Build history of the part. All positions in model axes, mm. A direction names the side the tool comes from. Coordinates: 2 decimals unless noted, no trailing zeros. Loops run counter-clockwise (first coordinate to the right, second up) from the corner with the lowest first, then second, coordinate; pieces in that order, holes last.
Item 1: Cut at B-B (x = -25). List the corners of the cut face in (y, z), and give its area (3 significant figures).
Item 2: Mould opens along Y. For faces 4 (the face through (-1, 4.5, 5)), 5 (the face through (92.5, 58.04, -0.16)), 6 (the face through (0, 98.1, -2)), 7 (the face through (-60.019, 87.575, -1.584)) say: released by +Y, released by -Y, zero draft, split by the parting line, or undercut.
Item 3: Cut at C-C (y = 65). List the corners of the cut face in (x, z).
Item 4: Cut at D-D (x = 60). List the corners of the cut face in (y, z), and give its area (3 significant figures).
Item 5: Drill centre lines: line 1 along Y through (x, z) = (36, -2.5); line 2 along X through (y, z) = (74, 4.25); line 3 along X through (y, z) = (64, -3.5). Where is each one in solid material? Low to high.
Item 6: Flat gauge pins, fed straight in: pin 1 (6 mm diameter, centred on x = 9, z = -3.5, fed in from -Y); pin 2 (4.5 mm diameter, centred on y = 60, z = -4.5, fed in from -X); pin 3 (3 mm diameter, centred on y = 86.5, z = 3.5, fed in from +X). Where does each tip first touch, or does it go through?
Item 7: 3-axis set-ups, long thin cutter, end or side, ignore diameter. For faces 1 (the face through (59.475, 88.119, -1.584)), 2 (the face through (0, 93.1, 0)), 3 (the face through (-78, 105, -7.5)): which of +Z, -Z, +X, -X, +Y, -Y reach the whole face in a straight line?
Item 8: Cut at A-A (z = 0). List the corners of the cut face in (x, y), and give its area (3 significant figures).
from build123d import *

# Parameters (mm, degrees)
BOSS_EXTRUDE1_DEPTH = 117.6
CUT_EXTRUDE4_DEPTH  = 12
CUT_EXTRUDE6_DEPTH  = 151.36957804
CUT_EXTRUDE7_DEPTH  = 4.5
CUT_EXTRUDE8_START  = 113.1
CUT_EXTRUDE8_DEPTH  = 4.5
CUT_EXTRUDE9_DEPTH  = 4.5
CUT_EXTRUDE10_START = 113.1
CUT_EXTRUDE10_DEPTH = 4.5


with BuildPart() as part:
    # Sketch2 → Boss-Extrude1 (new body)
    with BuildSketch(Plane(origin=(0, 0, 0), x_dir=(1, 0, 0), z_dir=(0, 1, 0))):
        with BuildLine():
            Line((85, -7.5), (-85, -7.5))
            ThreePointArc((-85, -7.5), (-92.5, 0), (-85, 7.5))
            Line((-85, 7.5), (85, 7.5))
            ThreePointArc((85, 7.5), (92.5, 0), (85, -7.5))
        make_face()
    extrude(amount=BOSS_EXTRUDE1_DEPTH)

    # Sketch3 → Cut-Extrude4 (cut)
    with BuildSketch(Plane(origin=(0, 0, -7.5), x_dir=(-1, 0, 0), z_dir=(0, 0, -1))):
        with BuildLine():
            Line((-50, 113.1), (50, 113.1))
            ThreePointArc((50, 113.1), (74.748737342, 102.848737342), (85, 78.1))
            Line((85, 78.1), (85, 39.5))
            ThreePointArc((85, 39.5), (74.748737342, 14.751262658), (50, 4.5))
            Line((50, 4.5), (-50, 4.5))
            ThreePointArc((-50, 4.5), (-74.748737342, 14.751262658), (-85, 39.5))
            Line((-85, 39.5), (-85, 78.1))
            ThreePointArc((-85, 78.1), (-74.748737342, 102.848737342), (-50, 113.1))
        make_face()
        with BuildLine():
            Line((-70, 63.1), (-70, 54.5))
            ThreePointArc((-70, 54.5), (-59.748737342, 29.751262658), (-35, 19.5))
            Line((-35, 19.5), (35, 19.5))
            ThreePointArc((35, 19.5), (59.748737342, 29.751262658), (70, 54.5))
            Line((70, 54.5), (70, 63.1))
            ThreePointArc((70, 63.1), (59.748737342, 87.848737342), (35, 98.1))
            Line((35, 98.1), (-35, 98.1))
            ThreePointArc((-35, 98.1), (-59.748737342, 87.848737342), (-70, 63.1))
        make_face(mode=Mode.SUBTRACT)
    extrude(amount=-CUT_EXTRUDE4_DEPTH, mode=Mode.SUBTRACT)

    # Sketch6 → Cut-Extrude6 (cut, through all)
    with BuildSketch(Plane(origin=(0, 0, -7.5), x_dir=(-1, 0, 0), z_dir=(0, 0, -1))):
        with BuildLine():
            Line((-35, 24.5), (35, 24.5))
            ThreePointArc((35, 24.5), (56.213203436, 33.286796564), (65, 54.5))
            Line((65, 54.5), (65, 63.1))
            ThreePointArc((65, 63.1), (56.213203436, 84.313203436), (35, 93.1))
            Line((35, 93.1), (-35, 93.1))
            ThreePointArc((-35, 93.1), (-56.213203436, 84.313203436), (-65, 63.1))
            Line((-65, 63.1), (-65, 54.5))
            ThreePointArc((-65, 54.5), (-56.213203436, 33.286796564), (-35, 24.5))
        make_face()
    extrude(amount=-CUT_EXTRUDE6_DEPTH, mode=Mode.SUBTRACT)

    # Sketch2_6 → Cut-Extrude7 (cut)
    with BuildSketch(Plane(origin=(0, 0, 0), x_dir=(1, 0, 0), z_dir=(0, 1, 0))):
        with BuildLine():
            Line((-8.2248772, -2.5), (8.2248772, -2.5))
            Line((8.2248772, -2.5), (15.34156858, -1.994983292))
            ThreePointArc((15.34156858, -1.994983292), (17.2, 0), (15.34156858, 1.994983292))
            Line((15.34156858, 1.994983292), (1.88348082, 2.95))
            ThreePointArc((1.88348082, 2.95), (0, 3.5), (-1.88348082, 2.95))
            Line((-1.88348082, 2.95), (-15.34156858, 1.994983292))
            ThreePointArc((-15.34156858, 1.994983292), (-17.2, 0), (-15.34156858, -1.994983292))
            Line((-15.34156858, -1.994983292), (-8.2248772, -2.5))
        make_face()
        with BuildLine():
            Line((1.88348082, -2.95), (8.2248772, -2.5))
            Line((8.2248772, -2.5), (-8.2248772, -2.5))
            Line((-8.2248772, -2.5), (-1.88348082, -2.95))
            ThreePointArc((-1.88348082, -2.95), (0, -3.5), (1.88348082, -2.95))
        make_face()
    extrude(amount=CUT_EXTRUDE7_DEPTH, mode=Mode.SUBTRACT)

    # Sketch2_7 → Cut-Extrude8 (cut)
    with BuildSketch(Plane(origin=(0, 0, 0), x_dir=(1, 0, 0), z_dir=(0, 1, 0)).offset(CUT_EXTRUDE8_START)):
        with BuildLine():
            Line((-8.2248772, -2.5), (8.2248772, -2.5))
            Line((8.2248772, -2.5), (15.34156858, -1.994983292))
            ThreePointArc((15.34156858, -1.994983292), (17.2, 0), (15.34156858, 1.994983292))
            Line((15.34156858, 1.994983292), (1.88348082, 2.95))
            ThreePointArc((1.88348082, 2.95), (0, 3.5), (-1.88348082, 2.95))
            Line((-1.88348082, 2.95), (-15.34156858, 1.994983292))
            ThreePointArc((-15.34156858, 1.994983292), (-17.2, 0), (-15.34156858, -1.994983292))
            Line((-15.34156858, -1.994983292), (-8.2248772, -2.5))
        make_face()
        with BuildLine():
            Line((1.88348082, -2.95), (8.2248772, -2.5))
            Line((8.2248772, -2.5), (-8.2248772, -2.5))
            Line((-8.2248772, -2.5), (-1.88348082, -2.95))
            ThreePointArc((-1.88348082, -2.95), (0, -3.5), (1.88348082, -2.95))
        make_face()
    extrude(amount=CUT_EXTRUDE8_DEPTH, mode=Mode.SUBTRACT)

    # Sketch2_8 → Cut-Extrude9 (cut)
    with BuildSketch(Plane(origin=(0, 0, 0), x_dir=(1, 0, 0), z_dir=(0, 1, 0))):
        with BuildLine():
            Line((85, -2.5), (85, 7.5))
            Line((85, 7.5), (-85, 7.5))
            Line((-85, 7.5), (-85, -2.5))
            Line((-85, -2.5), (-8.2248772, -2.5))
            Line((-8.2248772, -2.5), (-15.34156858, -1.994983292))
            ThreePointArc((-15.34156858, -1.994983292), (-17.2, 0), (-15.34156858, 1.994983292))
            Line((-15.34156858, 1.994983292), (-1.88348082, 2.95))
            ThreePointArc((-1.88348082, 2.95), (0, 3.5), (1.88348082, 2.95))
            Line((1.88348082, 2.95), (15.34156858, 1.994983292))
            ThreePointArc((15.34156858, 1.994983292), (17.2, 0), (15.34156858, -1.994983292))
            Line((15.34156858, -1.994983292), (8.2248772, -2.5))
            Line((8.2248772, -2.5), (85, -2.5))
        make_face()
        with BuildLine():
            Line((70, -7.5), (85, -7.5))
            ThreePointArc((85, -7.5), (92.5, 0), (85, 7.5))
            Line((85, 7.5), (85, -2.5))
            Line((85, -2.5), (8.2248772, -2.5))
            Line((8.2248772, -2.5), (1.88348082, -2.95))
            ThreePointArc((1.88348082, -2.95), (0, -3.5), (-1.88348082, -2.95))
            Line((-1.88348082, -2.95), (-8.2248772, -2.5))
            Line((-8.2248772, -2.5), (-85, -2.5))
            Line((-85, -2.5), (-85, 7.5))
            ThreePointArc((-85, 7.5), (-92.5, 0), (-85, -7.5))
            Line((-85, -7.5), (-70, -7.5))
            Line((-70, -7.5), (-55, -7.5))
            Line((-55, -7.5), (55, -7.5))
            Line((55, -7.5), (70, -7.5))
        make_face()
        with BuildLine():
            Line((1.88348082, -2.95), (8.2248772, -2.5))
            Line((8.2248772, -2.5), (-8.2248772, -2.5))
            Line((-8.2248772, -2.5), (-1.88348082, -2.95))
            ThreePointArc((-1.88348082, -2.95), (0, -3.5), (1.88348082, -2.95))
        make_face()
    extrude(amount=CUT_EXTRUDE9_DEPTH, mode=Mode.SUBTRACT)

    # Sketch2_9 → Cut-Extrude10 (cut)
    with BuildSketch(Plane(origin=(0, 0, 0), x_dir=(1, 0, 0), z_dir=(0, 1, 0)).offset(CUT_EXTRUDE10_START)):
        with BuildLine():
            Line((85, -2.5), (85, 7.5))
            Line((85, 7.5), (-85, 7.5))
            Line((-85, 7.5), (-85, -2.5))
            Line((-85, -2.5), (-8.2248772, -2.5))
            Line((-8.2248772, -2.5), (-15.34156858, -1.994983292))
            ThreePointArc((-15.34156858, -1.994983292), (-17.2, 0), (-15.34156858, 1.994983292))
            Line((-15.34156858, 1.994983292), (-1.88348082, 2.95))
            ThreePointArc((-1.88348082, 2.95), (0, 3.5), (1.88348082, 2.95))
            Line((1.88348082, 2.95), (15.34156858, 1.994983292))
            ThreePointArc((15.34156858, 1.994983292), (17.2, 0), (15.34156858, -1.994983292))
            Line((15.34156858, -1.994983292), (8.2248772, -2.5))
            Line((8.2248772, -2.5), (85, -2.5))
        make_face()
        with BuildLine():
            Line((70, -7.5), (85, -7.5))
            ThreePointArc((85, -7.5), (92.5, 0), (85, 7.5))
            Line((85, 7.5), (85, -2.5))
            Line((85, -2.5), (8.2248772, -2.5))
            Line((8.2248772, -2.5), (1.88348082, -2.95))
            ThreePointArc((1.88348082, -2.95), (0, -3.5), (-1.88348082, -2.95))
            Line((-1.88348082, -2.95), (-8.2248772, -2.5))
            Line((-8.2248772, -2.5), (-85, -2.5))
            Line((-85, -2.5), (-85, 7.5))
            ThreePointArc((-85, 7.5), (-92.5, 0), (-85, -7.5))
            Line((-85, -7.5), (-70, -7.5))
            Line((-70, -7.5), (-55, -7.5))
            Line((-55, -7.5), (55, -7.5))
            Line((55, -7.5), (70, -7.5))
        make_face()
        with BuildLine():
            Line((-8.2248772, -2.5), (8.2248772, -2.5))
            Line((8.2248772, -2.5), (15.34156858, -1.994983292))
            ThreePointArc((15.34156858, -1.994983292), (17.2, 0), (15.34156858, 1.994983292))
            Line((15.34156858, 1.994983292), (1.88348082, 2.95))
            ThreePointArc((1.88348082, 2.95), (0, 3.5), (-1.88348082, 2.95))
            Line((-1.88348082, 2.95), (-15.34156858, 1.994983292))
            ThreePointArc((-15.34156858, 1.994983292), (-17.2, 0), (-15.34156858, -1.994983292))
            Line((-15.34156858, -1.994983292), (-8.2248772, -2.5))
        make_face()
        with BuildLine():
            Line((1.88348082, -2.95), (8.2248772, -2.5))
            Line((8.2248772, -2.5), (-8.2248772, -2.5))
            Line((-8.2248772, -2.5), (-1.88348082, -2.95))
            ThreePointArc((-1.88348082, -2.95), (0, -3.5), (1.88348082, -2.95))
        make_face()
    extrude(amount=CUT_EXTRUDE10_DEPTH, mode=Mode.SUBTRACT)


solid = part.part
Filled sheet:
1. outline: (4.5, 4.5) - (19.5, 4.5) - (19.5, -7.5) - (24.5, -7.5) - (24.5, 7.5) - (4.5, 7.5) - close; (93.1, -7.5) - (98.1, -7.5) - (98.1, 4.5) - (113.1, 4.5) - (113.1, 7.5) - (93.1, 7.5) - close
1. area: 240 mm2
2. face 4: released by -Y
2. face 5: zero draft
2. face 6: released by +Y
2. face 7: undercut
3. outline: (-85, -7.5) - (-85, 4.5) - (-69.95, 4.5) - (-69.95, -7.5) - (-64.94, -7.5) - (-64.94, 7.5) - (-85, 7.5) arc R7.5 ccw to start; (64.94, -7.5) - (69.95, -7.5) - (69.95, 4.5) - (85, 4.5) - (85, -7.5) arc R7.5 ccw to (85, 7.5) - (64.94, 7.5) - close
4. outline: (4.5, -7.5) - (5.96, -7.5) - (5.96, 4.5) - (30.01, 4.5) - (30.01, -7.5) - (37.92, -7.5) - (37.92, 7.5) - (4.5, 7.5) - close; (79.68, -7.5) - (87.59, -7.5) - (87.59, 4.5) - (111.64, 4.5) - (111.64, -7.5) - (113.1, -7.5) - (113.1, 7.5) - (79.68, 7.5) - close
4. area: 425 mm2
5. line 1: y = 19.51 to 24.52, 93.08 to 98.09
5. line 2: x = -91.18 to -85, -68.26 to -62.95, 62.95 to 68.26, 85 to 91.18
5. line 3: x = -91.63 to -85, -69.99 to -64.99, 64.99 to 69.99, 85 to 91.63
6. pin 1: stops at y = 19.5
6. pin 2: stops at x = -92.15
6. pin 3: stops at x = 92.23
7. face 1: -Z
7. face 2: +Z, -Z
7. face 3: -Z, +X, -X, +Y, -Y
8. outline: (-92.5, 4.5) - (-50, 4.5) arc R35 cw to (-85, 39.5) - (-85, 78.1) arc R35 cw to (-50, 113.1) - (-92.5, 113.1) - close; (-70, 54.5) arc R35 ccw to (-35, 19.5) - (35, 19.5) arc R35 ccw to (70, 54.5) - (70, 63.1) arc R35 ccw to (35, 98.1) - (-35, 98.1) arc R35 ccw to (-70, 63.1) - close; (50, 4.5) - (92.5, 4.5) - (92.5, 113.1) - (50, 113.1) arc R35 cw to (85, 78.1) - (85, 39.5) arc R35 cw to start; hole (-65, 54.5) arc R30 ccw to (-35, 24.5) - (35, 24.5) arc R30 ccw to (65, 54.5) - (65, 63.1) arc R30 ccw to (35, 93.1) - (-35, 93.1) arc R30 ccw to (-65, 63.1) - close
8. area: 4,490 mm2
